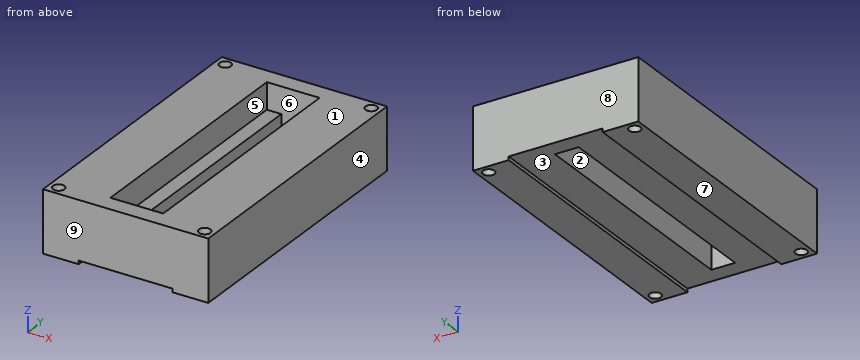
Autodesk Fusion 360 part; units mm, degrees
sketch "Sketch1" plane through (0, 0, 0) normal (0, 0, 1) x (1, 0, 0)
  line L0 (-23.5, 40) -> (23.5, 40)
  line L1 (23.5, 40) -> (23.5, -40)
  line L2 (23.5, -40) -> (-23.5, -40)
  line L3 (-23.5, -40) -> (-23.5, 40)
  line L4 (0, 40) -> (0, 0)
  line L5 (0, 0) -> (23.5, 0)
  line L6 (-20.75, 37.25) -> (-23.5, 37.25)
  line L7 (-20.75, -37.25) -> (-23.5, -37.25)
  line L8 (20.75, -37.25) -> (23.5, -37.25)
  line L9 (20.75, 37.25) -> (23.5, 37.25)
  line L10 (-20.75, 37.25) -> (-20.75, 40)
  line L11 (20.75, 37.25) -> (20.75, 40)
  line L12 (20.75, -37.25) -> (20.75, -40)
  line L13 (-20.75, -37.25) -> (-20.75, -40)
  point P0 (-20.75, 37.25)
  point P1 (20.75, 37.25)
  point P2 (20.75, -37.25)
  point P3 (-20.75, -37.25)
  dimension "d2" = 47
  dimension "d3" = 80
  dimension "d4" = 2.75
extrude "Extrude1" add sketch "Sketch1" along normal blind 17.5
hole "Hole1" at (-20.75, 37.25, 0) at (20.75, 37.25, 0) at (-20.75, -37.25, 0) at (20.75, -37.25, 0) direction (0, 0, 1) diameter 3.3 end through all
sketch "Sketch2" plane through (0, 0, 17.5) normal (0, 0, 1) x (-1, 0, 0)
  circle A0 centre (20.75, 37.25) radius 1.65
  circle A1 centre (20.75, -37.25) radius 1.65
  circle A2 centre (-20.75, -37.25) radius 1.65
  circle A3 centre (-20.75, 37.25) radius 1.65
  line L0 (23.5, 40) -> (-23.5, 40)
  line L1 (-23.5, 40) -> (-23.5, -40)
  line L2 (-23.5, -40) -> (23.5, -40)
  line L3 (23.5, -40) -> (23.5, 40)
  line L4 (0, 0) -> (-7.5, 0)
  line L5 (0, 0) -> (0, -35)
  line L6 (7.5, -35) -> (-7.5, -35)
  line L7 (-7.5, -35) -> (-7.5, 35)
  line L8 (-7.5, 35) -> (7.5, 35)
  line L9 (7.5, 35) -> (7.5, -35)
  dimension "d12" = 15
  dimension "d13" = 70
extrude "Extrude2" cut sketch "Sketch2" against normal blind 7.5 contours L4 L5 L6 L7 | L4 L5 L6 L7 L8 L9
sketch "Sketch3" plane through (0, 0, 10) normal (0, 0, 1) x (-1, 0, 0)
  line L0 (7.5, 35) -> (-7.5, 35)
  line L1 (-7.5, 35) -> (-7.5, -35)
  line L2 (-7.5, -35) -> (7.5, -35)
  line L3 (7.5, -35) -> (7.5, 35)
  line L4 (0, 0) -> (0, -35)
  line L5 (0, 0) -> (-3.375, 0)
  line L6 (3.375, -35) -> (-3.375, -35)
  line L7 (-3.375, -35) -> (-3.375, 35)
  line L8 (-3.375, 35) -> (3.375, 35)
  line L9 (3.375, 35) -> (3.375, -35)
  dimension "d16" = 70
  dimension "d17" = 6.75
extrude "Extrude3" cut sketch "Sketch3" against normal through all contours L0 L2 L4 L5 L6 L7 L8 L9 | L2 L4 L5 L6 L7
sketch "Sketch4" plane through (0, 0, 0) normal (0, 0, 1) x (1, 0, 0)
  line L0 (0, 0) -> (13.3476, 0)
  line L1 (0, 0) -> (0, -40)
  line L2 (-13.3476, -40) -> (13.3476, -40)
  line L3 (13.3476, -40) -> (13.3476, 40)
  line L4 (13.3476, 40) -> (-13.3476, 40)
  line L5 (-13.3476, 40) -> (-13.3476, -40)
extrude "Extrude4" cut sketch "Sketch4" along normal blind 1
For this review, take the finished solid that the model builds, in its own axes (mm). Face numbers are marked on the shaded views. A direction names the side the tool comes from. Coordinates: 2 decimals unless noted, no trailing zeros. Order: outer loops, then holes, each group sorted by start corner. A loop starts at its lowest first (then second) coordinate and runs counter-clockwise, first axis right, second up. Notation, with made-up numbers: (55, 83) -> (114, 83) arc R22 ccw to (114, 110) -> close; hole circle Ø3 at (54.25, -38.75). An arc over 180 degrees is marked (long way). Answer as CSV lines item,"result".
Q1. For the marked faces 1, 2, 3, 4 and 5, list the 3-axis set-ups (+Z, -Z, +X, -X, +Y, -Y) from which the entire face can be reached by the end or side of a thin tool; tool diameter is ignored.
Model answer:
face 1,"+Z, +X, -X, +Y, -Y"
face 2,"+Z, -Z"
face 3,"-Z, +Y, -Y"
face 4,"+Z, -Z, +X, +Y, -Y"
face 5,"+Z"
Q2. Draft analysis for pull direction Y (two halves, no side actions). For the marked faces 6, 7, 8 and 9, state which applies: released by +Y, released by -Y, zero draft, split by the parting line, or undercut.
Model answer:
face 6,"undercut"
face 7,"zero draft"
face 8,"released by +Y"
face 9,"released by -Y"
Q3. We need section B-B (z = 15.5). State the section outline as (x, y) points.
Model answer:
outline,"(-23.5, -40) -> (23.5, -40) -> (23.5, 40) -> (-23.5, 40) -> close; hole circle Ø3.3 at (-20.75, -37.25); hole circle Ø3.3 at (-20.75, 37.25); hole (-7.5, -35) -> (7.5, -35) -> (7.5, 35) -> (-7.5, 35) -> close; hole circle Ø3.3 at (20.75, -37.25); hole circle Ø3.3 at (20.75, 37.25)"
Q4. Clearance check with flat-ended pins moving along their axes: pin 1 Ø8 at (x, y) = (0.5, 8) entering from -Z; pin 2 Ø1.2 at (x, y) = (-5.5, 3) entering from +Z. State where each tip first meets the part, or that it passes through.
Model answer:
pin 1,"stops at z = 1"
pin 2,"stops at z = 10"
Q5. Wall thickness on line 1 along X through (y, z) = (37.25, 12.75); line 2 along Y through (x, z) = (20.75, 13); line 3 along X through (y, z) = (16, 7.75) (3 decimals): over which ranges is each line inside the solid? List them lowest first. Write a range as [from, to].
Model answer:
line 1,"x = [-23.5, -22.4], [-19.1, 19.1], [22.4, 23.5]"
line 2,"y = [-40, -38.9], [-35.6, 35.6], [38.9, 40]"
line 3,"x = [-23.5, -3.375], [3.375, 23.5]"
Q6. We need section C-C (y = -1.5). State the section outline as (x, z) points (3 decimals), plus the area to 3 significant figures.
Model answer:
outline,"(-23.5, 0) -> (-13.348, 0) -> (-13.348, 1) -> (-3.375, 1) -> (-3.375, 10) -> (-7.5, 10) -> (-7.5, 17.5) -> (-23.5, 17.5) -> close; (3.375, 1) -> (13.348, 1) -> (13.348, 0) -> (23.5, 0) -> (23.5, 17.5) -> (7.5, 17.5) -> (7.5, 10) -> (3.375, 10) -> close"
area,"623 mm2"
Q7. We need section D-D (x = -1). State the section outline as (y, z) points, plus the area to 3 significant figures.
Model answer:
outline,"(-40, 1) -> (-35, 1) -> (-35, 17.5) -> (-40, 17.5) -> close; (35, 1) -> (40, 1) -> (40, 17.5) -> (35, 17.5) -> close"
area,"165 mm2"
Q8. We need section A-A (x = 20.75). State the section outline as (y, z) points.
Model answer:
outline,"(-40, 0) -> (-38.9, 0) -> (-38.9, 17.5) -> (-40, 17.5) -> close; (-35.6, 0) -> (35.6, 0) -> (35.6, 17.5) -> (-35.6, 17.5) -> close; (38.9, 0) -> (40, 0) -> (40, 17.5) -> (38.9, 17.5) -> close"
